Geometry: see drawing. Coordinates: mm, zero at the bounding-box minimum. A direction names the side the tool comes from. Coordinates: 2 decimals unless noted, no trailing zeros. Loops run counter-clockwise (first coordinate to the right, second up) from the corner with the lowest first, then second, coordinate; pieces in that order, holes last. Notation, with made-up numbers: (-26.5, -18.75) - (3.5, -18.75) arc R15 ccw to (3.5, 6.25) - close; hole circle Ø6 at (40, 55). An arc over 180 degrees is marked (long way). Write each question's results on one line, items separated by ' | '. Start each with the question number.
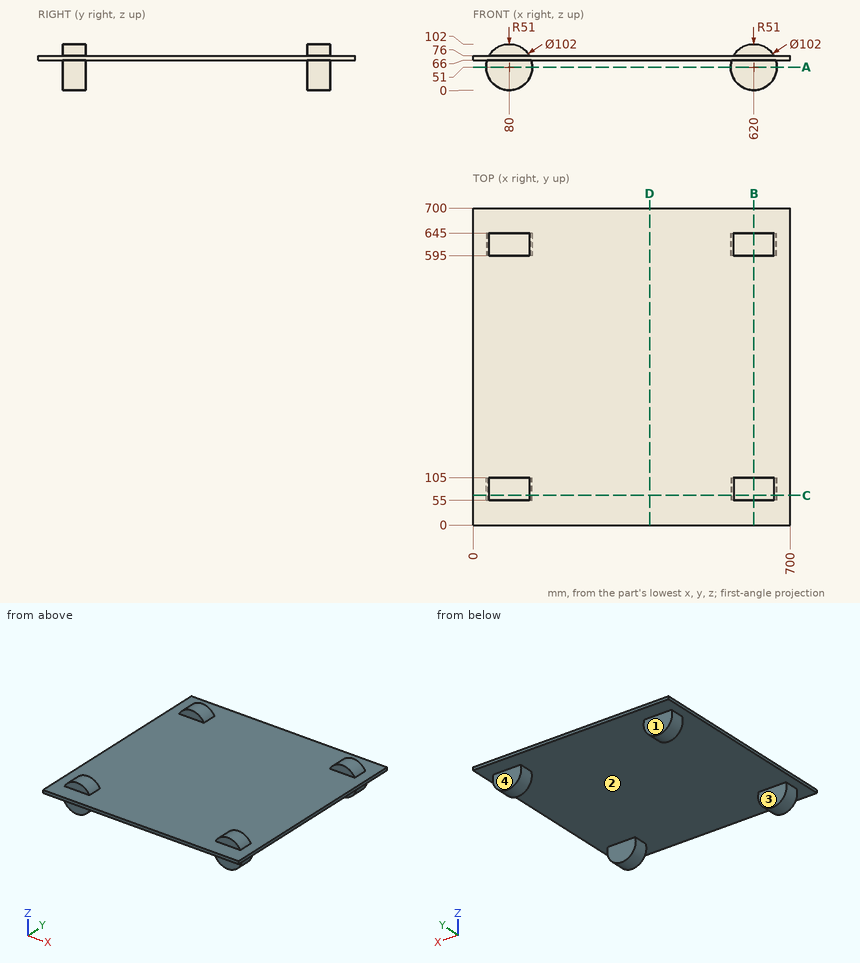
1) Section query A-A on z = 51. Output: boundary loops of the cut face in (x, y).
2) Material intervals for line 1 (X direction, y = 84, z = 26); line 2 (Z direction, x = 525.5, y = 246); line 3 (Y direction, x = 66.5, z = 41.5), sorted ascending. Write a range as [from, to].
3) Section query D-D on x = 390. Output: boundary loops of the cut face in (y, z).
4) Pin query (flat end, axial travel): pin 1 Ø13 at (x, z) = (634, 92.5) entering from +Y; pin 2 Ø13 at (x, z) = (97, 85) entering from -Y; pin 3 Ø6 at (x, y) = (214.5, 121.5) entering from -Z. Return the tip coordinate at first contact, or that it passes through.
5) Section query B-B on x = 620. Output: boundary loops of the cut face in (y, z), and give its area (3 significant figures).
6) Pull-direction query (Y, two-part tool) for the marked faces 1 and 2; classes: released by +Y, released by -Y, zero draft, split by the parting line, or undercut.
7) Section query C-C on y = 66. Output: boundary loops of the cut face in (x, z).
8) Access query for the marked faces 3 and 4. Directions: +Z, -Z, +X, -X, +Y, -Y. A direction counts if a zero-diameter tool reaches every point of the face in a straight line with its end or side. Return the directions, or none.
Returned:
1) outline: (29, 55) - (131, 55) - (131, 105) - (29, 105) - close; (29, 595) - (131, 595) - (131, 645) - (29, 645) - close; (569, 55) - (671, 55) - (671, 105) - (569, 105) - close; (569, 595) - (671, 595) - (671, 645) - (569, 645) - close
2) line 1: x = [35.55, 124.45], [575.55, 664.45] | line 2: z = [66, 76] | line 3: y = [55, 105], [595, 645]
3) outline: (0, 66) - (700, 66) - (700, 76) - (0, 76) - close
4) pin 1: stops at y = 645 | pin 2: stops at y = 55 | pin 3: stops at z = 66
5) outline: (0, 66) - (55, 66) - (55, 0) - (105, 0) - (105, 66) - (595, 66) - (595, 0) - (645, 0) - (645, 66) - (700, 66) - (700, 76) - (645, 76) - (645, 102) - (595, 102) - (595, 76) - (105, 76) - (105, 102) - (55, 102) - (55, 76) - (0, 76) - close | area: 16,200 mm²
6) face 1: released by +Y | face 2: undercut
7) outline: (0, 66) - (31.26, 66) arc R51 ccw (long way) to (128.74, 66) - (571.26, 66) arc R51 ccw (long way) to (668.74, 66) - (700, 66) - (700, 76) - (664.45, 76) arc R51 ccw to (575.55, 76) - (124.45, 76) arc R51 ccw to (35.55, 76) - (0, 76) - close
8) face 3: -Z, +X, -X | face 4: -Z, +X, -X, +Y
